```python
from build123d import *
from build123d import SkipClean  # not in build123d's __all__

# Parameters (mm, degrees)
F1_DEPTH  = 7
F2_DEPTH  = 33.02
F3_DEPTH  = 33.02
F4_DEPTH  = 33.02
F6_R      = 7.62
F5_R      = 11.25
F5_R_2    = 11
F7_DEPTH  = 25.4
F8_R      = 1.8749848785
F8_R_2    = 2.6443594024
F8_R_3    = 4.4059759684
F9_DEPTH  = 7
F10_R     = 1.27
F12_DEPTH = 25.4
F13_DEPTH = 7


with BuildPart() as f1:
    # F0 (on Top) → F1 (new body)
    with BuildSketch(Plane.XY):
        Polygon((14.2875, 8.248891971), (-14.2875, 8.248891971), (0, -16.4977839421), align=None)
    extrude(amount=F1_DEPTH)

    # F2 (add): a face of the model
    f2_faces = [f1.faces().sort_by_distance(p)[0] for p in [
        (-7.14375, -4.1244459855, 3.5),
    ]]
    extrude(f2_faces, amount=F2_DEPTH)

    # F3 (add): a face of the model
    f3_faces = [f1.faces().sort_by_distance(p)[0] for p in [
        (0, 8.248891971, 3.5),
    ]]
    extrude(f3_faces, amount=F3_DEPTH)

    # F4 (add): a face of the model
    f4_faces = [f1.faces().sort_by_distance(p)[0] for p in [
        (7.14375, -4.1244459855, 3.5),
    ]]
    extrude(f4_faces, amount=F4_DEPTH)

    # F6
    f6_edges = [f1.edges().sort_by_distance(p)[0] for p in [
        (-42.883659, -8.261108, 3.5),
        (-28.596159, -33.007784, 3.5),
        (28.596159, -33.007784, 3.5),
        (42.883659, -8.261108, 3.5),
        (14.2875, 41.268892, 3.5),
        (-14.2875, 41.268892, 3.5),
    ]]
    fillet(f6_edges, radius=F6_R)

    # F5 (on face) → F7 (cut)
    with BuildSketch(Plane.XY.offset(7)):
        with Locations((0, 27.298891971)):
            Circle(F5_R)
        Circle(F5_R_2)
        with BuildLine():
            ThreePointArc((34.8915339421, -13.6494459855), (12.7748683963, -10.7377317281), (33.3843197347, -19.2744459855))
            ThreePointArc((33.3843197347, -19.2744459855), (34.5081994878, -16.5611602429), (34.8915339421, -13.6494459855))
        make_face()
        with BuildLine():
            ThreePointArc((-12.3915339421, -13.6494459855), (-26.5532481995, -2.7827804398), (-33.3843197347, -19.2744459855))
            ThreePointArc((-33.3843197347, -19.2744459855), (-20.7298196847, -24.5161115313), (-12.3915339421, -13.6494459855))
        make_face()
    extrude(amount=-F7_DEPTH, mode=Mode.SUBTRACT)

    # F8 (on face) → F9 (join)
    with BuildSketch(Plane.XY.offset(7)):
        with BuildLine():
            ThreePointArc((-14.2875, 33.648891971), (-12.0556536726, 39.0370456437), (-6.6675, 41.268891971))
            ThreePointArc((-6.6675, 41.268891971), (-36.1939537613, 30.4970950948), (-51.8477511168, 3.2427063104))
            ThreePointArc((-51.8477511168, 3.2427063104), (-36.0457855424, 18.3806746008), (-14.2875, 16.048891971))
            Line((-14.2875, 16.048891971), (-14.2875, 33.648891971))
        make_face()
        with Locations((-40.1606029761, 21.0467017921)):
            Circle(F8_R, mode=Mode.SUBTRACT)
        with Locations((-32.5204535481, 26.0352350988)):
            Circle(F8_R_2, mode=Mode.SUBTRACT)
        with Locations((-21.5195283201, 28.9126522448)):
            Circle(F8_R_3, mode=Mode.SUBTRACT)
        with BuildLine():
            ThreePointArc((23.1156095166, -46.5228227514), (2.1047616282, -40.4069032795), (-6.7549981495, -20.3977839421))
            Line((-6.7549981495, -20.3977839421), (-21.9970452561, -29.1977839421))
            ThreePointArc((-21.9970452561, -29.1977839421), (-27.7792463798, -29.9590251616), (-32.406158833, -26.4086703653))
            ThreePointArc((-32.406158833, -26.4086703653), (-8.3142822131, -46.5934309681), (23.1156095166, -46.5228227514))
        make_face()
        with Locations((-6.286948215, -41.1811564646)):
            Circle(F8_R_2, mode=Mode.SUBTRACT)
        with Locations((-14.2793271748, -33.092784325)):
            Circle(F8_R_3, mode=Mode.SUBTRACT)
        with Locations((1.8533230702, -45.3034533047)):
            Circle(F8_R, mode=Mode.SUBTRACT)
        with BuildLine():
            Line((21.0424981495, 4.348891971), (21.3499965498, 4.1713576869))
            Line((21.3499965498, 4.1713576869), (36.2845452561, -4.451108029))
            ThreePointArc((36.2845452561, -4.451108029), (39.8349000524, -9.0780204821), (39.073658833, -14.8602216058))
            ThreePointArc((39.073658833, -14.8602216058), (44.5082359744, 16.0963358733), (28.7321416002, 43.280116441))
            ThreePointArc((28.7321416002, 43.280116441), (33.9410239142, 22.0262286786), (21.0424981495, 4.348891971))
        make_face()
        with Locations((35.7988554948, 4.1801320802)):
            Circle(F8_R_3, mode=Mode.SUBTRACT)
        with Locations((38.8074017631, 15.1459213658)):
            Circle(F8_R_2, mode=Mode.SUBTRACT)
        with Locations((38.3072799059, 24.2567515126)):
            Circle(F8_R, mode=Mode.SUBTRACT)
    extrude(amount=-F9_DEPTH)

    # F10
    f10_edges = [f1.edges().sort_by_distance(p)[0] for p in [
        (28.732142, 43.280116, 3.5),
        (23.11561, -46.522823, 3.5),
        (-51.847751, 3.242706, 3.5),
    ]]
    fillet(f10_edges, radius=F10_R)

    # F11 (on face) → F12 (cut)
    with BuildSketch(Plane.XY.offset(7)):
        with BuildLine():
            ThreePointArc((-15.7584187023, 4.4480611953), (-15.7224513331, 6.0815584331), (-15.3052551523, 7.6612907599))
            Line((-15.3052551523, 7.6612907599), (-21.0424981495, 4.348891971))
            ThreePointArc((-21.0424981495, 4.348891971), (-19.2958492313, 4.5353251977), (-17.9847825572, 3.3662897117))
            ThreePointArc((-17.9847825572, 3.3662897117), (-17.8870097802, 3.2797249828), (-17.7572116819, 3.2940575304))
            Line((-17.7572116819, 3.2940575304), (-15.7584187023, 4.4480611953))
        make_face()
        with BuildLine():
            ThreePointArc((-11.9076836854, 13.8921337202), (-13.5756314513, 14.443033023), (-14.2875, 16.048891971))
            Line((-14.2875, 16.048891971), (-14.2875, 9.4240943934))
            ThreePointArc((-14.2875, 9.4240943934), (-13.1280097642, 10.5752630477), (-11.7313433439, 11.423160322))
            Line((-11.7313433439, 11.423160322), (-11.7313433439, 13.7311676517))
            ThreePointArc((-11.7313433439, 13.7311676517), (-11.7838300426, 13.850742376), (-11.9076836854, 13.8921337202))
        make_face()
        with BuildLine():
            ThreePointArc((-6.0770988718, -17.2584234319), (-5.72021778, -18.9783582208), (-6.7549981495, -20.3977839421))
            Line((-6.7549981495, -20.3977839421), (-1.0177551523, -17.0853851533))
            ThreePointArc((-1.0177551523, -17.0853851533), (-2.5944415689, -16.6568214807), (-4.0270753584, -15.8712215173))
            Line((-4.0270753584, -15.8712215173), (-6.0258683381, -17.0252251822))
            ThreePointArc((-6.0258683381, -17.0252251822), (-6.1031797376, -17.1304673587), (-6.0770988718, -17.2584234319))
        make_face()
        with BuildLine():
            ThreePointArc((4.0270753584, -15.8712215173), (2.5944415689, -16.6568214807), (1.0177551523, -17.0853851533))
            Line((1.0177551523, -17.0853851533), (6.7549981495, -20.3977839421))
            ThreePointArc((6.7549981495, -20.3977839421), (5.72021778, -18.9783582208), (6.0770988718, -17.2584234319))
            ThreePointArc((6.0770988718, -17.2584234319), (6.1031797376, -17.1304673587), (6.0258683381, -17.0252251822))
            Line((6.0258683381, -17.0252251822), (4.0270753584, -15.8712215173))
        make_face()
        with BuildLine():
            Line((21.0424981495, 4.348891971), (15.3052551523, 7.6612907599))
            ThreePointArc((15.3052551523, 7.6612907599), (15.7224513331, 6.0815584331), (15.7584187023, 4.4480611953))
            Line((15.7584187023, 4.4480611953), (17.7572116819, 3.2940575304))
            ThreePointArc((17.7572116819, 3.2940575304), (17.8870097802, 3.2797249828), (17.9847825572, 3.3662897117))
            ThreePointArc((17.9847825572, 3.3662897117), (19.2958492313, 4.5353251977), (21.0424981495, 4.348891971))
        make_face()
        with BuildLine():
            Line((14.2875, 9.4240943934), (14.2875, 16.048891971))
            ThreePointArc((14.2875, 16.048891971), (13.5756314513, 14.443033023), (11.9076836854, 13.8921337202))
            ThreePointArc((11.9076836854, 13.8921337202), (11.7838300426, 13.850742376), (11.7313433439, 13.7311676517))
            Line((11.7313433439, 13.7311676517), (11.7313433439, 11.423160322))
            ThreePointArc((11.7313433439, 11.423160322), (13.1280097642, 10.5752630477), (14.2875, 9.4240943934))
        make_face()
    extrude(amount=-F12_DEPTH, mode=Mode.SUBTRACT)

    # F11 (on face) → F13 (join)
    with BuildSketch(Plane.XY.offset(7)):
        with BuildLine():
            Line((-14.2875, 8.248891971), (-14.2875, 9.4240943934))
            ThreePointArc((-14.2875, 9.4240943934), (-14.8614145652, 8.5802416998), (-15.3052551523, 7.6612907599))
            Line((-15.3052551523, 7.6612907599), (-14.2875, 8.248891971))
        make_face()
        with BuildLine():
            Line((0, -16.4977839421), (-1.0177551523, -17.0853851533))
            ThreePointArc((-1.0177551523, -17.0853851533), (0, -17.1604833996), (1.0177551523, -17.0853851533))
            Line((1.0177551523, -17.0853851533), (0, -16.4977839421))
        make_face()
        with BuildLine():
            ThreePointArc((15.3052551523, 7.6612907599), (14.8614145652, 8.5802416998), (14.2875, 9.4240943934))
            Line((14.2875, 9.4240943934), (14.2875, 8.248891971))
            Line((14.2875, 8.248891971), (15.3052551523, 7.6612907599))
        make_face()
    with SkipClean():  # cleaning this boolean's faces spoils the solid; the shape is the same uncleaned
        extrude(amount=-F13_DEPTH)


solid = f1.part
```
Geometry: final body of the model. Coordinates: model frame, mm. A direction names the side the tool comes from. Coordinates: 2 decimals unless noted, no trailing zeros. Order: outer loops, then holes, each group sorted by start corner. A loop starts at its lowest first (then second) coordinate and runs counter-clockwise, first axis right, second up. Notation, with made-up numbers: (-5, 10) - (46, 10) arc R22 cw to (46, 36) - close; hole circle Ø9 at (64.25, 16). An arc over 180 degrees is marked (long way). Write each question's results on one line, items separated by ' | '.
(1) Section query B-B, the plane y = -35.5. Return the cut outline in (x, z), plus the area to 3 significant figures.
Values found:
outline: (-25.52, 0) - (-17.97, 0) - (-17.97, 7) - (-25.52, 7) - close; (-10.59, 0) - (-2.25, 0) - (-2.25, 7) - (-10.59, 7) - close | area: 111 mm²
(2) Section query A-A, the plane y = -7.5. Return the cut outline in (x, z), plus the area to 3 significant figures.
Values found:
outline: (-39.22, 0) - (-33.06, 0) - (-33.06, 7) - (-39.22, 7) - close; (-14.22, 0) - (-8.05, 0) - (-8.05, 7) - (-14.22, 7) - close; (8.05, 0) - (14.22, 0) - (14.22, 7) - (8.05, 7) - close; (33.06, 0) - (42.49, 0) - (42.49, 7) - (33.06, 7) - close | area: 196 mm²
(3) Mould query, pull axis X, two halves, no side actions, for faces 1 (the face through (0.47, -44.04, 3.55)), 2 (the face through (-6, 10, 7)), 3 (the face through (-5.715, -18.954, 3.549)), 4 (the face through (-28.56, 0.01, 3.45)). Classes: +X half, -X half, draft (parallel to the pull), parting line (faces both ways), or undercut.
Values found:
face 1: undercut | face 2: draft | face 3: undercut | face 4: -X half
(4) Set-up query: faces 5 (the face through (-39.856, -9.159, 3.549)), 6 (the face through (11.731, 13, 4)), 7 (the face through (14.288, 25, 3)). Return all of +Z, -Z, +X, -X, +Y, -Y with unobstructed straight access to the full face (end or side cutting, diameter ignored); none if empty.
Values found:
face 5: +Z, -Z, -X | face 6: +Z, -Z | face 7: +Z, -Z, +Y
(5) Section query D-D, the plane z = 2.5. Count the separate pieces of the cut face and the enclosed holes in it, plus the area to 3 significant figures.
Values found:
separate pieces: 1 | enclosed holes: 13 | area: 2,740 mm²
(6) Section query C-C, the plane x = -23.5. Return the cut outline in (y, z).
Values found:
outline: (-37.45, 0) - (-24.9, 0) - (-24.9, 7) - (-37.45, 7) - close; (-2.4, 0) - (2.93, 0) - (2.93, 7) - (-2.4, 7) - close; (19.43, 0) - (24.98, 0) - (24.98, 7) - (19.43, 7) - close; (32.85, 0) - (38.07, 0) - (38.07, 7) - (32.85, 7) - close
(7) First-contact query: pin 1 Ø0.7 at (y, z) = (13, 3) entering from +X; pin 2 Ø20 at (x, y) = (0, 0) entering from -Z; pin 3 Ø4 at (x, z) = (20, 1.5) entering from +Y. Flat tips, straight axial feed; report the tip coordinate or a pass-through.
Values found:
pin 1: stops at x = 44.99 | pin 2: passes through | pin 3: stops at y = 4.91
(8) Line query: line 1 (X direction, y = -23, z = 5.5); line 2 (X direction, y = 16, z = 3.5); line 3 (Y direction, x = -17.5, z = 1.25). Output: solid intervals per line, ascending. Write a range as [from, to].
Values found:
line 1: x = [-34.37, -29.9], [-17.39, -6.67], [11.26, 17.39], [29.9, 34.37] | line 2: x = [-47.64, -41.14], [-14.29, 14.29], [31.96, 36.3], [41.31, 44.53] | line 3: y = [-42.05, -36.1], [-30.09, -23.08], [-4.22, 3.44], [17.69, 27.11], [30.72, 39.97]
